Part model, mm, in its own coordinate system. A direction names the side the tool comes from. Give positions to 0.01 mm unless a question says otherwise; leave off trailing zeros. Write each loop counter-clockwise with the first axis right and the second up, starting at its lowest first coordinate (ties: lowest second). Pieces come first, ordered by that corner, then holes.
from build123d import *

# Parameters (mm, degrees)
SKETCH1_R           = 6.5
BOSS_EXTRUDE1_DEPTH = 18
SKETCH2_R           = 5
CUT_EXTRUDE1_DEPTH  = 4
CUT_EXTRUDE2_DEPTH  = 12
CHAMFER1_SIZE       = 1
CHAMFER1_SIZE2      = 0.577350269
SKETCH4_OUTSIDE_W   = 20.146
SKETCH4_OUTSIDE_H   = 20.146
SKETCH4_OUTSIDE_R   = 5.5
CUT_EXTRUDE3_DEPTH  = 15
CHAMFER2_SIZE       = 15
CHAMFER2_SIZE_2     = 0.786116689


with BuildPart() as part:
    # Sketch1 → Boss-Extrude1 (new body)
    with BuildSketch(Plane(origin=(0, 0, 0), x_dir=(1, 0, 0), z_dir=(0, 1, 0))):
        with Locations(Location((0, 0, 0), (0, 0, 270))):
            Circle(SKETCH1_R)
    extrude(amount=BOSS_EXTRUDE1_DEPTH)

    # Sketch2 → Cut-Extrude1 (cut)
    with BuildSketch(Plane.XZ):
        with Locations(Location((0, 0, 0), (0, 0, 270))):
            Circle(SKETCH2_R)
    extrude(amount=-CUT_EXTRUDE1_DEPTH, mode=Mode.SUBTRACT)

    # Sketch3 → Cut-Extrude2 (cut)
    with BuildSketch(Plane.XZ.offset(-4)):
        with BuildLine():
            Line((-1.732055507, -2.57098886), (3.04828024, -0.563903873))
            ThreePointArc((3.04828024, -0.563903873), (-1.200087257, 2.858284551), (-1.732055507, -2.57098886))
        make_face()
    extrude(amount=-CUT_EXTRUDE2_DEPTH, mode=Mode.SUBTRACT)

    # Chamfer1
    chamfer1_edges = [part.edges().sort_by_distance(p)[0] for p in [
        (0, 0, 5),
    ]]
    chamfer1_side = [part.faces().sort_by_distance(p)[0] for p in [
        (0, 2, 5),
    ]]
    chamfer(chamfer1_edges, length=CHAMFER1_SIZE, length2=CHAMFER1_SIZE2, reference=chamfer1_side[0])

    # Sketch4 outside → Cut-Extrude3 (cut)
    with BuildSketch(Plane(origin=(0, 18, 0), x_dir=(1, 0, 0), z_dir=(0, 1, 0))):
        Rectangle(SKETCH4_OUTSIDE_W, SKETCH4_OUTSIDE_H)
        with Locations(Location((0, 0, 0), (0, 0, 270))):
            Circle(SKETCH4_OUTSIDE_R, mode=Mode.SUBTRACT)
    extrude(amount=-CUT_EXTRUDE3_DEPTH, mode=Mode.SUBTRACT)

    # Chamfer2
    # the kernel refuses this chamfer: 15, 0.786116689 mm, written as the material it takes off along each edge
    with BuildSketch(Plane(origin=(0, 18, 0), x_dir=(0, 0, 1), z_dir=(-1, 0, 0))) as chamfer2_piece_1_section:
        Polygon((5.5, -CHAMFER2_SIZE), (5.5 - CHAMFER2_SIZE_2, 0), (5.5, 0), align=None)
    chamfer2_piece_1 = revolve(axis=Axis((0, 18, 0), (0, 1, 0)), mode=Mode.PRIVATE)
    chamfer2_piece_1 = split(chamfer2_piece_1, bisect_by=Plane(origin=(0, 3, -5.162730795), z_dir=(0, 1, 0)), keep=Keep.TOP, mode=Mode.PRIVATE)
    add(chamfer2_piece_1, mode=Mode.SUBTRACT)


solid = part.part
1) Flat gauge pins, fed straight in: P1, Ø5, axis at x = -1.5, z = 0.5, coming from the -Y side; P2, Ø1.5, axis at x = -1.5, y = 16, coming from the -Z side; P3, Ø3, axis at x = 4.5, y = 12.5, coming from the +Z side. Where does each tip first touch, or does it go through?
Check result:
P1: stops at y = 4
P2: stops at z = -4.77
P3: stops at z = 4.01
2) Saw through at B-B (x = 0). Write the cut outline in (y, z).
Check result:
outline: (0, -6.5) - (3, -6.5) - (3, -5.5) - (18, -4.71) - (18, 4.71) - (3, 5.5) - (3, 6.5) - (0, 6.5) - (0, 5.58) - (1, 5) - (4, 5) - (4, 3.1) - (16, 3.1) - (16, -1.84) - (4, -1.84) - (4, -5) - (1, -5) - (0, -5.58) - close
3) Mould opens along Z. For faces 1 (the cylindrical face through (-3.955, 1.479, -5.158)), 2 (the flat face through (0, 18, 0)), 3 (the flat face through (0.1, 4, -2.2)) say: +Z half, -Z half, draft (parallel to the pull), parting line (faces both ways), or undercut.
Check result:
face 1: parting line
face 2: draft
face 3: undercut
4) Saw through at C-C (y = 6.5). Write the cut outline in (x, z), and give its area (3 significant figures).
Check result:
outline: circle Ø10.63 at (0, 0); hole (-1.73, -2.57) - (3.05, -0.56) arc R3.1 ccw (long way) to start
area: 63.7 mm2
5) 3-axis set-ups, long thin cutter, end or side, ignore diameter. For faces 4 (the cylindrical face through (-1.1, 9.9, 2.9)), 5 (the flat face through (5, 0, 3)), 6 (the flat face through (-5, 3, -3)): which of +Z, -Z, +X, -X, +Y, -Y reach the whole face in a straight line?
Check result:
face 4: -Y
face 5: +Z, -Z, +X, -X, -Y
face 6: +Y
6) Drill centre lines: L1, parallel to X at y = 2, z = 0; L2, parallel to Z at x = 0, y = 9; L3, parallel to Y at x = -3, z = 0.5. Where is each one in solid material? Low to high.
Check result:
L1: x = -6.5 to -5, 5 to 6.5
L2: z = -5.19 to -1.84, 3.1 to 5.19
L3: y = 16 to 18
7) Saw through at A-A (z = 0). Write the cut outline in (x, y).
Check result:
outline: (-6.5, 0) - (-5.58, 0) - (-5, 1) - (-5, 4) - (-3.1, 4) - (-3.1, 16) - (3.1, 16) - (3.1, 4) - (5, 4) - (5, 1) - (5.58, 0) - (6.5, 0) - (6.5, 3) - (5.5, 3) - (4.71, 18) - (-4.71, 18) - (-5.5, 3) - (-6.5, 3) - close
8) Saw through at D-D (y = 13.75). Write the cut outline in (x, z).
Check result:
outline: circle Ø9.87 at (0, 0); hole (-1.73, -2.57) - (3.05, -0.56) arc R3.1 ccw (long way) to start
